Design review of the part built by this model. Coordinates are the model's own, in mm. A direction names the side the tool comes from. Give positions to 0.01 mm unless a question says otherwise; leave off trailing zeros. Loops run counter-clockwise (first coordinate to the right, second up) from the corner with the lowest first, then second, coordinate; pieces in that order, holes last.
from build123d import *

# Parameters (mm, degrees)
EXTRUDE_1_DEPTH     = 45.4
EXTRUDE_START       = -6.5
EXTRUDE_2_DEPTH     = 32.4
CHAMFER_1_SIZE      = 0.5
SKETCH_3_R          = 1.5
CUT_EXTRUDE_1_DEPTH = 3.5


with BuildPart() as part:
    # 草图1 → 凸台-拉伸1 (new body)
    with BuildSketch(Plane.XY):
        Polygon((-13.5, 0), (13.5, 0), (13.5, -10), (6, -10), (6, -6), (-6, -6), (-6, -10), (-13.5, -10), align=None)
    extrude(amount=EXTRUDE_1_DEPTH)

    # 草图2 → 凸台-拉伸2 (add)
    with BuildSketch(Plane.XY.offset(45.4).offset(EXTRUDE_START)):
        Polygon((14, -10), (14, 0.5), (-14, 0.5), (-14, -10), (-13.5, -10), (-13.5, 0), (13.5, 0), (13.5, -10), align=None)
    extrude(amount=-EXTRUDE_2_DEPTH)

    # 倒角1
    chamfer_1_edges = [part.edges().sort_by_distance(p)[0] for p in [
        (13.5, -10, 42.15),
        (6, -10, 22.7),
        (6, -6, 22.7),
        (-6, -6, 22.7),
        (-6, -10, 22.7),
        (-13.5, -10, 42.15),
        (-13.5, 0, 42.15),
        (13.5, 0, 42.15),
        (13.5, -10, 3.25),
        (-13.5, -10, 3.25),
        (-13.5, 0, 3.25),
        (13.5, 0, 3.25),
    ]]
    chamfer(chamfer_1_edges, length=CHAMFER_1_SIZE)

    # 草图3 → 切除-拉伸1 (cut)
    with BuildSketch(Plane(origin=(0, 0.5, 0), x_dir=(1, 0, 0), z_dir=(0, 1, 0))):
        with Locations(Location((10, -12.7, 0), (0, 0, 270))):
            Circle(SKETCH_3_R)
        with Locations(Location((10, -32.7, 0), (0, 0, 90))):
            Circle(SKETCH_3_R)
        with Locations(Location((-10, -32.7, 0), (0, 0, 270))):
            Circle(SKETCH_3_R)
        with Locations(Location((-10, -12.7, 0), (0, 0, 90))):
            Circle(SKETCH_3_R)
    extrude(amount=-CUT_EXTRUDE_1_DEPTH, mode=Mode.SUBTRACT)


solid = part.part
Q1. Tool access review of faces 1 (the face through (-13.5, -5, 42)), 2 (the face through (-9.425, -1.226, 11.314)), 3 (the face through (13.5, -5, 3)), 4 (the face through (-6, -8, 22)): name each direction out of +Z, -Z, +X, -X, +Y, -Y from which nothing blocks a thin tool from reaching the whole face with its end or side.
Results:
face 1: +Z, -X, +Y, -Y
face 2: +Y
face 3: -Z, +X, +Y, -Y
face 4: +Z, -Z, -Y
Q2. Draft analysis for pull direction X (two halves, no side actions). For faces 5 (the face through (-10, -10, 22)), 6 (the face through (10, -3, 13)), 7 (the face through (-14, -5, 23)), state which applies: pulls with the +X half, pulls with the -X half, needs draft (parallel to the pull), parting line crosses it, or undercut.
Results:
face 5: needs draft
face 6: undercut
face 7: pulls with the -X half
Q3. Insertion check: pin 1 (5 mm diameter, centred on y = -3, z = 41.5, fed in from +X); pin 2 (0.9 mm diameter, centred on x = -10, z = 33, fed in from +Y); pin 3 (7 mm diameter, centred on x = 5, z = 3.5, fed in from +Y); pin 4 (3.5 mm diameter, centred on x = 1.5, z = 20.5, fed in from -Y). Each pin has a flat end and moves straight along its axis. Give the tip position at first contact, or say it passes through.
Results:
pin 1: stops at x = 13.5
pin 2: stops at y = -3
pin 3: stops at y = 0.5
pin 4: stops at y = -6
Q4. Wall thickness on line 1 (X direction, y = -0.95, z = 12.7); line 2 (X direction, y = -8.75, z = 11); line 3 (Y direction, x = 4.5, z = 7.5): over which ranges is each line inside the solid? List them lowest first.
Results:
line 1: x = -14 to -11.5, -8.5 to 8.5, 11.5 to 14
line 2: x = -14 to -6, 6 to 14
line 3: y = -6 to 0.5
Q5. Take a section at B-B (x = -10). Give the boundary of the cut face in (y, z), plus the area to 3 significant figures.
Results:
outline: (-10, 0) - (0, 0) - (0, 6.5) - (0.5, 6.5) - (0.5, 11.2) - (-3, 11.2) - (-3, 14.2) - (0.5, 14.2) - (0.5, 31.2) - (-3, 31.2) - (-3, 34.2) - (0.5, 34.2) - (0.5, 38.9) - (0, 38.9) - (0, 45.4) - (-10, 45.4) - close
area: 449 mm2
Q6. Take a section at D-D (x = 5). Give the boundary of the cut face in (y, z).
Results:
outline: (-6, 0) - (0, 0) - (0, 6.5) - (0.5, 6.5) - (0.5, 38.9) - (0, 38.9) - (0, 45.4) - (-6, 45.4) - close
Q7. Take a section at A-A (y = -2.25). Give the boundary of the cut face in (x, z).
Results:
outline: (-14, 6.5) - (-13.5, 6.5) - (-13.5, 0) - (13.5, 0) - (13.5, 6.5) - (14, 6.5) - (14, 38.9) - (13.5, 38.9) - (13.5, 45.4) - (-13.5, 45.4) - (-13.5, 38.9) - (-14, 38.9) - close; hole circle Ø3 at (-10, 12.7); hole circle Ø3 at (-10, 32.7); hole circle Ø3 at (10, 12.7); hole circle Ø3 at (10, 32.7)
Q8. Take a section at C-C (z = 8.5). Give the boundary of the cut face in (x, y).
Results:
outline: (-14, -10) - (-6.5, -10) - (-6, -9.5) - (-6, -6.5) - (-5.5, -6) - (5.5, -6) - (6, -6.5) - (6, -9.5) - (6.5, -10) - (14, -10) - (14, 0.5) - (-14, 0.5) - close
